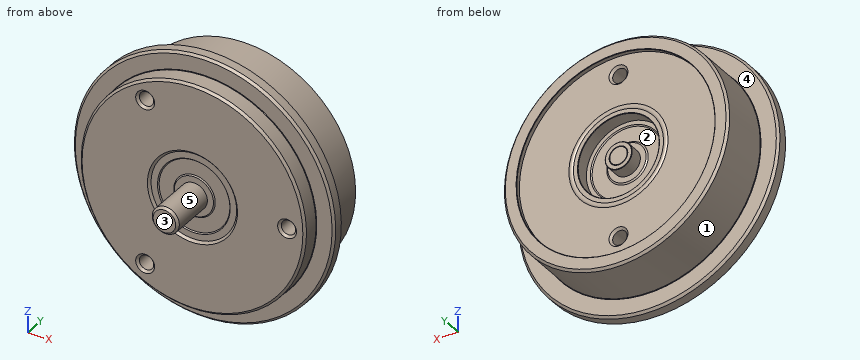
```python
from build123d import *

# Parameters (mm, degrees)
SKETCH2_R          = 1.6
CUT_EXTRUDE1_DEPTH = 6
SKETCH4_R          = 1.6
CUT_EXTRUDE2_DEPTH = 6
CHAMFER3_SIZE      = 0.1
CHAMFER1_SIZE      = 0.5


with BuildPart() as part:
    # Sketch1 → Revolve4 (revolve)
    with BuildSketch(Plane.XY, mode=Mode.PRIVATE) as revolve4_sk:
        with BuildLine():
            Line((840.942387276, 295.38888375), (840.051505549, 295.38888375))
            Line((840.051505549, 295.38888375), (839.795142101, 295.163855609))
            Line((839.795142101, 295.163855609), (836.54874871, 295.163855609))
            Line((836.54874871, 295.163855609), (836.207694111, 295.38888375))
            Line((836.207694111, 295.38888375), (834.942387276, 295.38888375))
            Line((834.942387276, 295.38888375), (834.942387276, 298.38888375))
            Line((834.942387276, 298.38888375), (834.009912561, 298.38888375))
            Line((834.009912561, 298.38888375), (833.942387276, 298.320272963))
            Line((833.942387276, 298.320272963), (833.872673537, 298.38888375))
            Line((833.872673537, 298.38888375), (831.942387276, 298.38888375))
            Line((831.942387276, 298.38888375), (831.942387276, 270.88888375))
            Line((831.942387276, 270.88888375), (834.942387276, 270.88888375))
            Line((834.942387276, 270.88888375), (834.942387276, 281.38888375))
            Line((834.942387276, 281.38888375), (836.2976122, 281.38888375))
            Line((836.2976122, 281.38888375), (836.54874871, 281.619976989))
            Line((836.54874871, 281.619976989), (839.795142101, 281.619976989))
            Line((839.795142101, 281.619976989), (840.007791728, 281.38888375))
            Line((840.007791728, 281.38888375), (841.442387276, 281.38888375))
            Line((841.442387276, 281.38888375), (841.942387276, 280.88888375))
            Line((841.942387276, 280.88888375), (856.942387276, 280.88888375))
            Line((856.942387276, 280.88888375), (856.942387276, 284.88888375))
            Line((856.942387276, 284.88888375), (860.942387276, 284.88888375))
            Line((860.942387276, 284.88888375), (860.942387276, 287.88888375))
            Line((860.942387276, 287.88888375), (856.942387276, 287.88888375))
            Line((856.942387276, 287.88888375), (856.942387276, 299.38888375))
            Line((856.942387276, 299.38888375), (853.942387276, 299.38888375))
            Line((853.942387276, 299.38888375), (853.942387276, 298.38888375))
            Line((853.942387276, 298.38888375), (842.942387276, 298.38888375))
            ThreePointArc((842.942387276, 298.38888375), (842.442387276, 298.595990531), (841.942387276, 298.38888375))
            Line((841.942387276, 298.38888375), (840.942387276, 298.38888375))
            Line((840.942387276, 298.38888375), (840.942387276, 295.38888375))
        make_face()
    revolve(revolve4_sk.sketch.rotate(Axis((831.942387276, 300.670444461, 0), (0, -1, 0)), 90), axis=Axis((831.942387276, 300.670444461, 0), (0, -1, 0)))

    # Sketch2 → Cut-Extrude1 (cut)
    with BuildSketch(Plane(origin=(0, 298.38888375, 0), x_dir=(-1, 0, 0), z_dir=(0, 1, 0))):
        with Locations(Location((-831.939085095, 17.999999697, 0), (0, 0, 90))):
            Circle(SKETCH2_R)
        with Locations(Location((-831.939085095, -17.999999697, 0), (0, 0, 90))):
            Circle(SKETCH2_R)
    extrude(amount=-CUT_EXTRUDE1_DEPTH, mode=Mode.SUBTRACT)

    # Sketch4 → Cut-Extrude2 (cut)
    with BuildSketch(Plane.XZ.offset(-280.88888375)):
        with Locations(Location((852.942387276, 0, 0), (0, 0, 270))):
            Circle(SKETCH4_R)
        with Locations(Location((821.442387276, -18.186533479, 0), (0, 0, 270))):
            Circle(SKETCH4_R)
        with Locations(Location((821.442387276, 18.186533479, 0), (0, 0, 270))):
            Circle(SKETCH4_R)
    extrude(amount=-CUT_EXTRUDE2_DEPTH, mode=Mode.SUBTRACT)

    # Cut-Extrude3 cone 1 section (through the dimple's axis) → Cut-Extrude3 (revolve, cut)
    with BuildSketch(Plane(origin=(831.939085095, 292.38888375, 17.999999697), x_dir=(0, 0, 1), z_dir=(1, 0, 0))):
        Polygon((0, 0), (1.6, 0), (0, 1.120332061), align=None)
    revolve(axis=Axis((831.939085095, 292.38888375, 17.999999697), (0, -1, 0)), mode=Mode.SUBTRACT)

    # Cut-Extrude3 cone 2 section (through the dimple's axis) → Cut-Extrude3 cone 2 (revolve, cut)
    with BuildSketch(Plane(origin=(831.939085095, 292.38888375, -17.999999697), x_dir=(0, 0, 1), z_dir=(1, 0, 0))):
        Polygon((0, 0), (1.6, 0), (0, 1.120332061), align=None)
    revolve(axis=Axis((831.939085095, 292.38888375, -17.999999697), (0, -1, 0)), mode=Mode.SUBTRACT)

    # Cut-Extrude4 cone 1 section (through the dimple's axis) → Cut-Extrude4 (revolve, cut)
    with BuildSketch(Plane(origin=(821.442387276, 286.88888375, 18.186533479), x_dir=(0, 0, -1), z_dir=(1, 0, 0))):
        Polygon((0, 0), (1.6, 0), (0, 1.120332061), align=None)
    revolve(axis=Axis((821.442387276, 286.88888375, 18.186533479), (0, 1, 0)), mode=Mode.SUBTRACT)

    # Cut-Extrude4 cone 2 section (through the dimple's axis) → Cut-Extrude4 cone 2 (revolve, cut)
    with BuildSketch(Plane(origin=(821.442387276, 286.88888375, -18.186533479), x_dir=(0, 0, -1), z_dir=(1, 0, 0))):
        Polygon((0, 0), (1.6, 0), (0, 1.120332061), align=None)
    revolve(axis=Axis((821.442387276, 286.88888375, -18.186533479), (0, 1, 0)), mode=Mode.SUBTRACT)

    # Cut-Extrude4 cone 3 section (through the dimple's axis) → Cut-Extrude4 cone 3 (revolve, cut)
    with BuildSketch(Plane(origin=(852.942387276, 286.88888375, 0), x_dir=(0, 0, -1), z_dir=(1, 0, 0))):
        Polygon((0, 0), (1.6, 0), (0, 1.120332061), align=None)
    revolve(axis=Axis((852.942387276, 286.88888375, 0), (0, 1, 0)), mode=Mode.SUBTRACT)

    # Chamfer3
    chamfer3_edges = [part.edges().sort_by_distance(p)[0] for p in [
        (831.942387276, 298.38888375, -3),
        (831.942387276, 284.88888375, -25),
        (831.942387276, 287.88888375, -25),
        (831.942387276, 299.38888375, -22),
        (831.942387276, 298.38888375, -9),
    ]]
    chamfer(chamfer3_edges, length=CHAMFER3_SIZE)

    # Chamfer1
    chamfer1_edges = [part.edges().sort_by_distance(p)[0] for p in [
        (831.942387276, 270.88888375, -3),
        (831.942387276, 280.88888375, -25),
        (831.942387276, 284.88888375, -29),
        (831.942387276, 287.88888375, -29),
        (831.942387276, 299.38888375, -25),
        (831.939085095, 298.38888375, 16.399999697),
        (831.939085095, 298.38888375, -19.599999697),
        (852.942387276, 280.88888375, 1.6),
        (821.442387276, 280.88888375, -16.586533479),
        (821.442387276, 280.88888375, 19.786533479),
    ]]
    chamfer(chamfer1_edges, length=CHAMFER1_SIZE)


solid = part.part
```
CAD build for the part. Positions are in the model's coordinates, mm. Face numbers are marked on the shaded views. A direction names the side the tool comes from. Give positions to 0.01 mm unless a question says otherwise; leave off trailing zeros. Loops run counter-clockwise (first coordinate to the right, second up) from the corner with the lowest first, then second, coordinate; pieces in that order, holes last. Notation, with made-up numbers: (11.5, -11) -> (57.5, -11) arc R19 ccw to (57.5, 26) -> close; hole circle Ø11 at (-2, -6). An arc over 180 degrees is marked (long way). Use a Markdown table: item, result.
1. Mould opens along Z. For the marked faces 1, 2 and 3 say: pulls with the +Z half, pulls with the -Z half, needs draft (parallel to the pull), parting line crosses it, or undercut.
Check result:
| item | result |
|---|---|
| face 1 | parting line crosses it |
| face 2 | undercut |
| face 3 | needs draft |
2. Flat gauge pins, fed straight in: pin 1 (2.5 mm diameter, centred on x = 831.5, z = -2, fed in from +Y); pin 2 (22 mm diameter, centred on x = 831.5, z = -9, fed in from +Y); pin 3 (1.5 mm diameter, centred on x = 821.5, z = -6, fed in from -Y). Where does each tip first touch, or does it go through?
Check result:
| item | result |
|---|---|
| pin 1 | stops at y = 298.39 |
| pin 2 | stops at y = 298.6 |
| pin 3 | stops at y = 280.89 |
3. Wall check: L1, parallel to X at y = 283.05, z = 0; L2, parallel to Y at x = 845, z = 10; L3, parallel to Y at x = 832.5, z = -7. Give the ranges that are in metal, low to high. Write a range as [from, to].
Check result:
| item | result |
|---|---|
| L1 | x = [806.94, 851.34], [854.54, 856.94] |
| L2 | y = [280.89, 298.39] |
| L3 | y = [281.62, 295.16] |
4. Slice it at A-A (y = 278.5). List the corners of the cut face in (x, z).
Check result:
| item | result |
|---|---|
| outline | circle Ø6 at (831.94, 0) |
5. Slice it at B-B (y = 289). List the corners of the cut face in (x, z), plus the area to 3 significant figures.
Check result:
| item | result |
|---|---|
| outline | circle Ø50 at (831.94, 0) |
| area | 1,960 mm^2 |
6. Which spindle directions (+Z, -Z, +X, -X, +Y, -Y) get a long thin tool onto all of the face, cutting with end or side? Do the marked faces 4 and 5. Say none if no direction does.
Check result:
| item | result |
|---|---|
| face 4 | +Y |
| face 5 | -Y |
